Geometry: see drawing. Coordinates: mm, zero at the bounding-box minimum. Give positions to 0.01 mm unless a question says otherwise; leave off trailing zeros. Loops run counter-clockwise (first coordinate to the right, second up) from the corner with the lowest first, then second, coordinate; pieces in that order, holes last. Notation, with made-up numbers: M -40,5 L -26,5 A11 cw -26,10 Z; hole C 67,2 d4. An arc over 180 degrees is marked long. Answer in a Markdown table with one row per item.
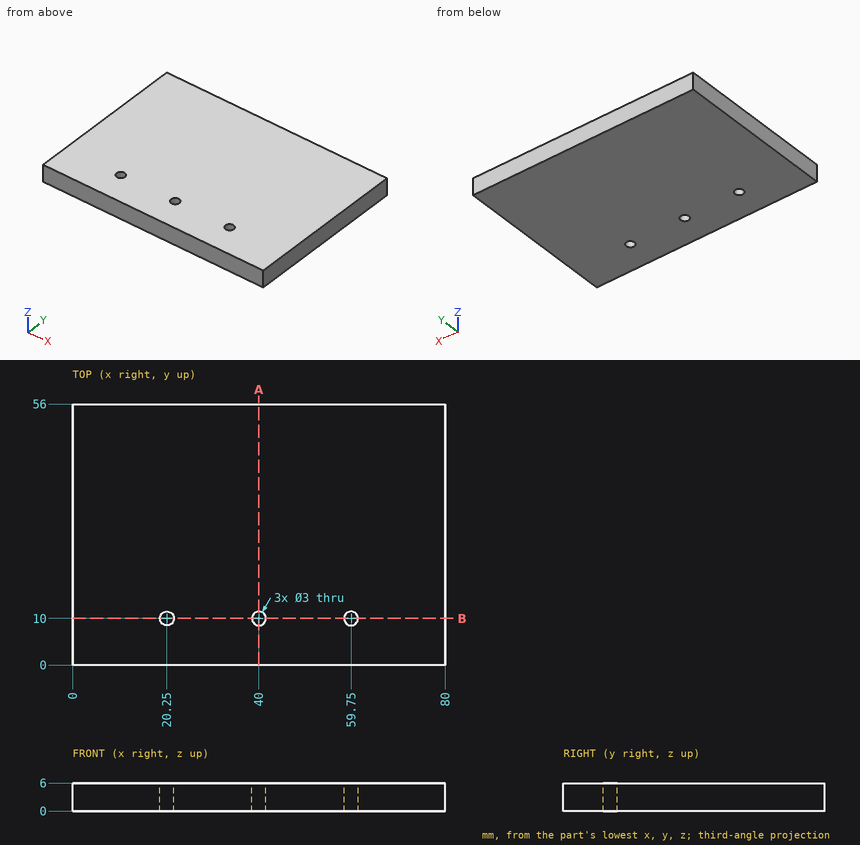
1) Section B-B, the plane y = 10. Return loops of the section in (x, z).
Reply:
| item | result |
|---|---|
| outline | M 0,0 L 18.75,0 L 18.75,6 L 0,6 Z; M 21.75,0 L 38.5,0 L 38.5,6 L 21.75,6 Z; M 41.5,0 L 58.25,0 L 58.25,6 L 41.5,6 Z; M 61.25,0 L 80,0 L 80,6 L 61.25,6 Z |
2) Section A-A, the plane x = 40. Return loops of the section in (y, z), then the cut area to 3 significant figures.
Reply:
| item | result |
|---|---|
| outline | M 0,0 L 8.5,0 L 8.5,6 L 0,6 Z; M 11.5,0 L 56,0 L 56,6 L 11.5,6 Z |
| area | 318 mm² |
3) Material intervals for L1, parallel to X at y = 10, z = 4.75; L2, parallel to Y at x = 40, z = 3.15; L3, parallel to Y at x = 58.5, z = 3.9, sorted ascending.
Reply:
| item | result |
|---|---|
| L1 | x = 0 to 18.75, 21.75 to 38.5, 41.5 to 58.25, 61.25 to 80 |
| L2 | y = 0 to 8.5, 11.5 to 56 |
| L3 | y = 0 to 9.17, 10.83 to 56 |
